Answer from the drawing. Dimensions are ordinates in mm from the lowest x, y and z of the part. A direction names the side the tool comes from. Coordinates: 2 decimals unless noted, no trailing zeros. Loops run counter-clockwise (first coordinate to the right, second up) from the corner with the lowest first, then second, coordinate; pieces in that order, holes last. Notation, with made-up numbers: (64.5, 77) -> (74.5, 77) arc R31 ccw to (74.5, 107) -> close; hole circle Ø10 at (3, 76). An arc over 180 degrees is marked (long way). Use a Markdown table: item, result.
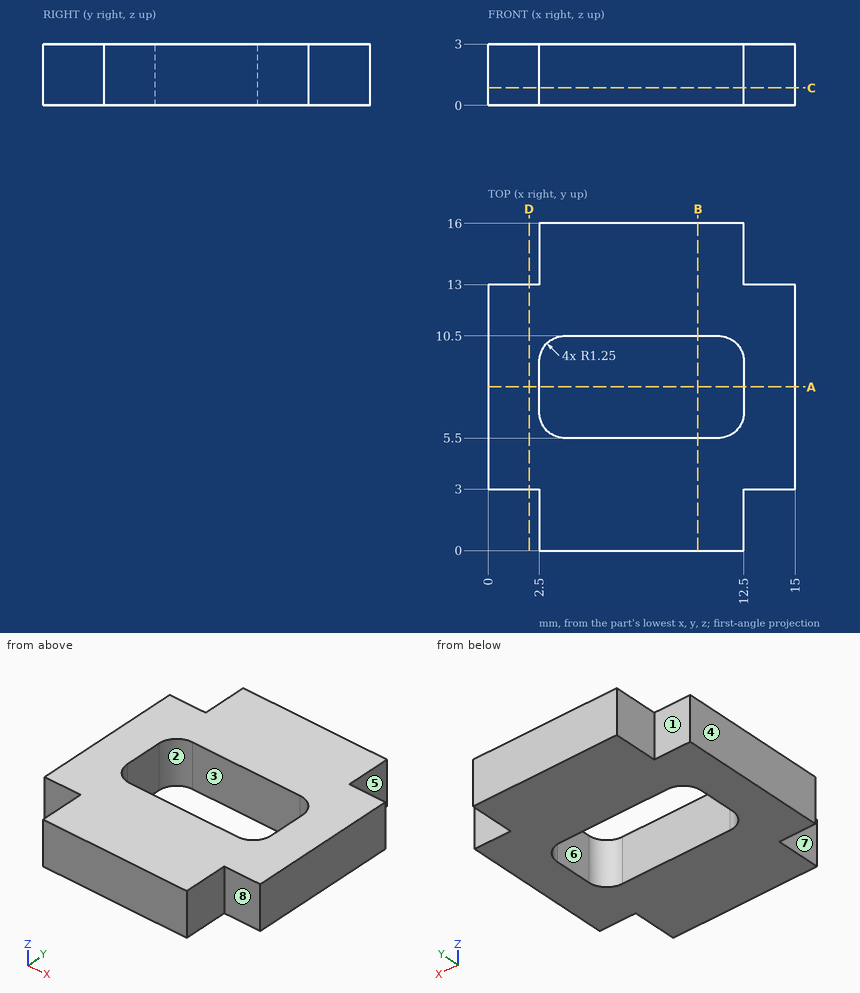
Q1. Section A-A on y = 8 is taken. Determine the outline of the cut face in (x, z).
Solved:
| item | result |
|---|---|
| outline | (0, 0) -> (2.5, 0) -> (2.5, 3) -> (0, 3) -> close; (12.5, 0) -> (15, 0) -> (15, 3) -> (12.5, 3) -> close |
Q2. For the marked faces 5, 6, 7 and 8, determine the directions among +Z, -Z, +X, -X, +Y, -Y from which every point of the face is accessible in a straight line to the end or side of a thin tool.
Solved:
| item | result |
|---|---|
| face 5 | +Z, -Z, +X, +Y |
| face 6 | +Z, -Z |
| face 7 | +Z, -Z, -X, -Y |
| face 8 | +Z, -Z, +X, -Y |
Q3. Section D-D on x = 2 is taken. Determine the outline of the cut face in (y, z), and give its area (3 significant figures).
Solved:
| item | result |
|---|---|
| outline | (3, 0) -> (13, 0) -> (13, 3) -> (3, 3) -> close |
| area | 30.0 mm² |
Q4. Determine the mould class of the marked faces 1, 2, 3 and 4 for opening direction X: pulls with the +X half, pulls with the -X half, needs draft (parallel to the pull), parting line crosses it, or undercut.
Solved:
| item | result |
|---|---|
| face 1 | needs draft |
| face 2 | undercut |
| face 3 | undercut |
| face 4 | pulls with the -X half |
Q5. Section B-B on x = 10.25 is taken. Determine the outline of the cut face in (y, z).
Solved:
| item | result |
|---|---|
| outline | (0, 0) -> (5.5, 0) -> (5.5, 3) -> (0, 3) -> close; (10.5, 0) -> (16, 0) -> (16, 3) -> (10.5, 3) -> close |
Q6. Section C-C on z = 0.85 is taken. Determine the outline of the cut face in (x, y), and give its area (3 significant figures).
Solved:
| item | result |
|---|---|
| outline | (0, 3) -> (2.5, 3) -> (2.5, 0) -> (12.5, 0) -> (12.5, 3) -> (15, 3) -> (15, 13) -> (12.5, 13) -> (12.5, 16) -> (2.5, 16) -> (2.5, 13) -> (0, 13) -> close; hole (2.5, 6.75) arc R1.25 ccw to (3.75, 5.5) -> (11.25, 5.5) arc R1.25 ccw to (12.5, 6.75) -> (12.5, 9.25) arc R1.25 ccw to (11.25, 10.5) -> (3.75, 10.5) arc R1.25 ccw to (2.5, 9.25) -> close |
| area | 161 mm² |
Q7. Consider line 1 (Y direction, x = 7.75, z = 1.8); line 2 (X direction, y = 7, z = 2.5); line 3 (X direction, y = 10.25, z = 1.95). Determine where each line is inside the solid, lowest interval first. Write a range as [from, to].
Solved:
| item | result |
|---|---|
| line 1 | [0, 5.5], [10.5, 16] |
| line 2 | [0, 2.5], [12.5, 15] |
| line 3 | [0, 3], [12, 15] |
Q8. Given pin 1 Ø1.5 at (x, y) = (4.5, 3.5) entering from -Z; pin 2 Ø0.8 at (x, z) = (14, 2) entering from +Y; pin 3 Ø0.9 at (y, z) = (15, 1) entering from +X, each flat-ended and moving along its own axis, determine where each tip first touches the part or whether it passes through.
Solved:
| item | result |
|---|---|
| pin 1 | z = 0 |
| pin 2 | y = 13 |
| pin 3 | x = 12.5 |
